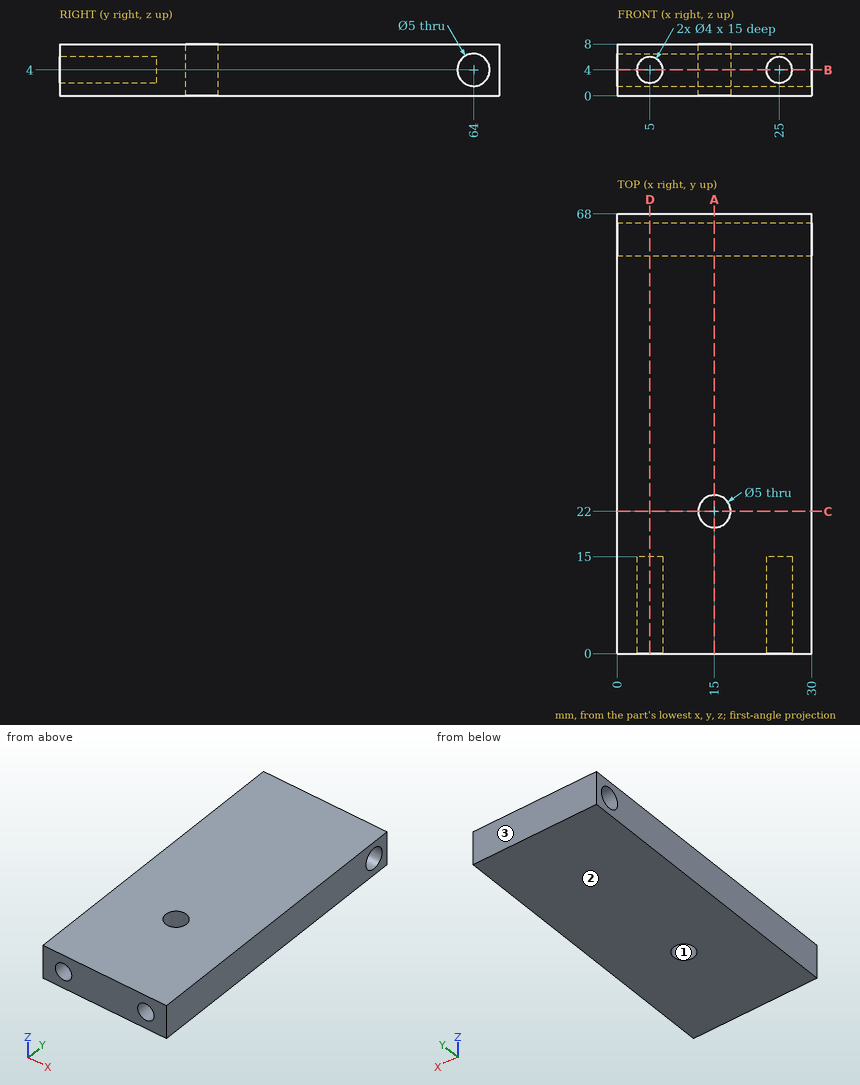
Check sheet for the drawn part. Datum: minimum x, y, z corner. Units: mm. Give positions to 0.01 mm unless a question says otherwise; leave off trailing zeros. Order: outer loops, then holes, each group sorted by start corner. A loop starts at its lowest first (then second) coordinate and runs counter-clockwise, first axis right, second up. Notation, with made-up numbers: (-33.5, 87) -> (0.5, 87) arc R22 ccw to (0.5, 126) -> close; hole circle Ø9 at (54.25, -4). An arc over 180 degrees is marked (long way). Return JSON: item names as keys, results as strings.
1. Cross-section at A-A, the plane x = 15. Record the cut outline in (y, z), plus the area to 3 significant figures.
From the geometry:
{"outline": "(0, 0) -> (19.5, 0) -> (19.5, 8) -> (0, 8) -> close; (24.5, 0) -> (68, 0) -> (68, 8) -> (24.5, 8) -> close; hole circle Ø5 at (64, 4)", "area": "484 mm^2"}
2. Material ranges on probe 1 along X at (y, z) = (10, 4); probe 2 along Y at (x, z) = (15, 3.75); probe 3 along Z at (x, y) = (18, 64), recorded low to high. Write a range as [from, to].
From the geometry:
{"probe 1": "[0, 3], [7, 23], [27, 30]", "probe 2": "[0, 19.5], [24.5, 61.51], [66.49, 68]", "probe 3": "[0, 1.5], [6.5, 8]"}
3. Go/stop test with a flat-tipped pin: P1, Ø2, axis at x = 5.5, z = 4, coming from the -Y side. Record where the tip stops, or that it passes through.
From the geometry:
{"P1": "y = 15"}
4. Cross-section at B-B, the plane z = 4. Record the cut outline in (x, y), plus the area to 3 significant figures.
From the geometry:
{"outline": "(0, 0) -> (3, 0) -> (3, 15) -> (7, 15) -> (7, 0) -> (23, 0) -> (23, 15) -> (27, 15) -> (27, 0) -> (30, 0) -> (30, 61.5) -> (0, 61.5) -> close; (0, 66.5) -> (30, 66.5) -> (30, 68) -> (0, 68) -> close; hole circle Ø5 at (15, 22)", "area": "1,750 mm^2"}
5. Cross-section at D-D, the plane x = 5. Record the cut outline in (y, z).
From the geometry:
{"outline": "(0, 0) -> (68, 0) -> (68, 8) -> (0, 8) -> (0, 6) -> (15, 6) -> (15, 2) -> (0, 2) -> close; hole circle Ø5 at (64, 4)"}
6. Cross-section at C-C, the plane y = 22. Record the cut outline in (x, z).
From the geometry:
{"outline": "(0, 0) -> (12.5, 0) -> (12.5, 8) -> (0, 8) -> close; (17.5, 0) -> (30, 0) -> (30, 8) -> (17.5, 8) -> close"}
7. Mould release check, pull along Y, two halves, no side actions. Record for the marked faces 1, 2 and 3: +Y half, -Y half, draft (parallel to the pull), parting line (faces both ways), or undercut.
From the geometry:
{"face 1": "undercut", "face 2": "draft", "face 3": "+Y half"}
